Could you check a few things on this drawing? It's one solid part, dimensions in mm from its lowest x, y, z. Give positions to 0.01 mm unless a question says otherwise; leave off trailing zeros. Loops run counter-clockwise (first coordinate to the right, second up) from the corner with the lowest first, then second, coordinate; pieces in that order, holes last. Notation, with made-up numbers: (-36.5, -18.5) - (-4.5, -18.5) arc R19 cw to (-4.5, -9.5) - close; hole circle Ø1 at (15.25, 6). An arc over 180 degrees is marked (long way). Write item = value, one per line.
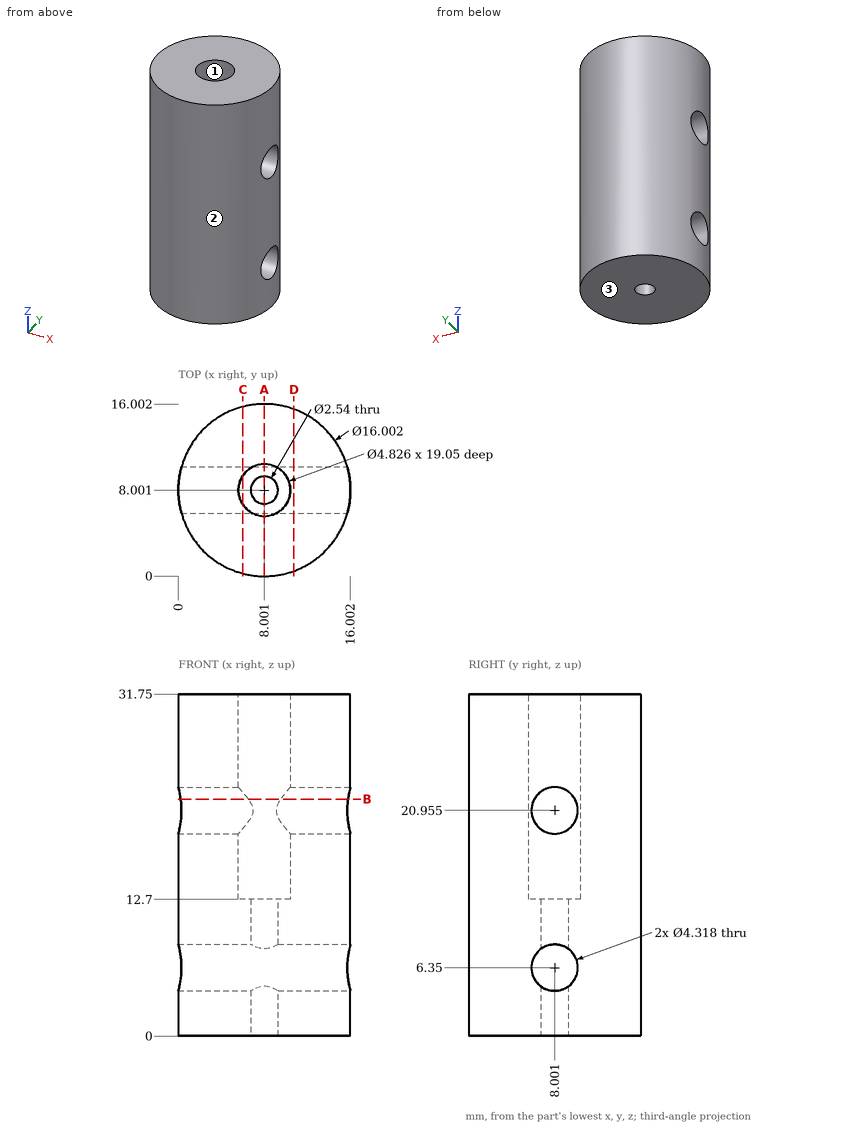
Q1. Imagine slicing it at B-B, the plane z = 22. Write out the boundary of the cut face in (x, y).
Output:
outline = (0.23, 6.11) arc R8 ccw to (15.78, 6.11) - (9.5, 6.11) arc R2.41 cw to (6.5, 6.11) - close; (0.23, 9.89) - (6.5, 9.89) arc R2.41 cw to (9.5, 9.89) - (15.78, 9.89) arc R8 ccw to start
Q2. Imagine slicing it at D-D, the plane x = 10.75. Write out the boundary of the cut face in (y, z) (3 decimals).
Output:
outline = (0.487, 0) - (15.515, 0) - (15.515, 31.75) - (0.487, 31.75) - close; hole circle Ø4.318 at (8.001, 6.35); hole circle Ø4.318 at (8.001, 20.955)
Q3. For pin 1 (6 mm diameter, centred on x = 3, z = 26, fed in from -Y); pin 2 (4 mm diameter, centred on x = 8.001, y = 8.001, fed in from +Z); pin 3 (1 mm diameter, centred on y = 14, z = 7.5, fed in from +X); pin 4 (5.5 mm diameter, centred on y = 8.001, z = 20.955, fed in from -X), each with a flat end and sliding along its axis, tell me the tip position at first contact or that it passes through.
Output:
pin_1 = 0.25
pin_2 = 12.7
pin_3 = 13.81
pin_4 = 0
Q4. I need wall thicknesses on L1, parallel to Z at x = 1.5, y = 8; L2, parallel to Z at x = 9.75, y = 9.75; L3, parallel to Y at x = 6.75, z = 26.5. Which ranges of each line are inside material? Lowest first, please.
Output:
L1 = 0 to 4.19, 8.51 to 18.8, 23.11 to 31.75
L2 = 0 to 5.08, 7.62 to 19.69, 22.22 to 31.75
L3 = 0.1 to 5.94, 10.06 to 15.9
Q5. We'd pull the mould along X, two halves only. Please class the marked faces 1, 2 and 3: released by +X, released by -X, zero draft, split by the parting line, or undercut.
Output:
face_1 = undercut
face_2 = split by the parting line
face_3 = zero draft
Q6. Imagine slicing it at A-A, the plane x = 8. Write out the boundary of the cut face in (y, z), then the cut area to 3 significant figures.
Output:
outline = (0, 0) - (6.73, 0) - (6.73, 4.6) arc R2.16 cw to (6.73, 8.1) - (6.73, 12.7) - (5.59, 12.7) - (5.59, 31.75) - (0, 31.75) - close; (9.27, 0) - (16, 0) - (16, 31.75) - (10.41, 31.75) - (10.41, 12.7) - (9.27, 12.7) - (9.27, 8.1) arc R2.16 cw to (9.27, 4.6) - close
area = 380 mm2
Q7. Imagine slicing it at C-C, the plane x = 6. Write out the boundary of the cut face in (y, z) (3 decimals), then the cut area to 3 significant figures.
Output:
outline = (0.254, 0) - (15.748, 0) - (15.748, 31.75) - (9.35, 31.75) - (9.35, 22.641) arc R2.159 cw to (9.35, 19.269) - (9.35, 12.7) - (6.652, 12.7) - (6.652, 19.269) arc R2.159 cw to (6.652, 22.641) - (6.652, 31.75) - (0.254, 31.75) - close; hole circle Ø4.318 at (8.001, 6.35)
area = 422 mm2
